Source: CAD feature listing. Evaluate the final solid. Frame: model axes, mm. A direction names the side the tool comes from. Round coordinates to 2 decimals unless told otherwise and drop trailing zeros. Order: outer loops, then holes, each group sorted by start corner. A loop starts at its lowest first (then second) coordinate and runs counter-clockwise, first axis right, second up. Notation, with made-up numbers: (56.25, -27.75) -> (105.25, -27.75) arc R28 ccw to (105.25, 11.25) -> close; hole circle Ø7 at (15, 47.5). An arc over 180 degrees is marked (long way). Answer as CSV lines item,"result".
from build123d import *

# Parameters (mm, degrees)
F2_SIZE2 = 1.3
F2_SIZE  = 0.8
F3_R     = 1.4
F4_SIZE2 = 0.5
F4_SIZE  = 2
F5_R     = 0.5


with BuildPart() as f1:
    # F0 (on Front) → F1 (revolve)
    with BuildSketch(Plane.XZ):
        Polygon((-24.5, 0), (-28.5, 0), (-28.5, -2), (-25, -2), (-25, -11), (-24.1, -11), (-24.1, -4), (-23.226406, -4), (-22.813906, -5.5), (-21.9, -5.5), (-23, -1.5), (-24.5, -1.5), align=None)
    revolve(axis=Axis((0, 0, 1.068981), (0, 0, -1)))

    # F2
    f2_edges = [f1.edges().sort_by_distance(p)[0] for p in [
        (28.5, 0, 0),
    ]]
    chamfer(f2_edges, length=F2_SIZE, length2=F2_SIZE2)

    # F3
    f3_edges = [f1.edges().sort_by_distance(p)[0] for p in [
        (25, 0, -2),
    ]]
    fillet(f3_edges, radius=F3_R)

    # F4
    f4_edges = [f1.edges().sort_by_distance(p)[0] for p in [
        (25, 0, -11),
    ]]
    chamfer(f4_edges, length=F4_SIZE, length2=F4_SIZE2)

    # F5
    f5_edges = [f1.edges().sort_by_distance(p)[0] for p in [
        (23.226406, 0, -4),
    ]]
    fillet(f5_edges, radius=F5_R)


solid = f1.part
1. Reachability of faces 4 (the cylindrical face through (-13.17, 20.66, -0.74)), 5 (the flat face through (-16.22, -18.03, -11)), 6 (the cylindrical face through (17.76, 16.29, -7.45)) from +Z, -Z, +X, -X, +Y, -Y: full face, straight path, thin tool, end or side. Return the list, or none.
Results below:
face 4,"+Z"
face 5,"-Z, +X, -X, +Y, -Y"
face 6,"-Z"
2. Mould query, pull axis X, two halves, no side actions, for faces 1 (the cylindrical face through (-23.846, 7.509, -6.239)), 2 (the flat face through (8.6, 20.4, -5.5)), 3 (the flat face through (-19, -19, -2)). Classes: released by +X, released by -X, zero draft, split by the parting line, or undercut.
Results below:
face 1,"split by the parting line"
face 2,"undercut"
face 3,"zero draft"
3. Section query C-C on z = -7.75. Return loops of the section in (x, y).
Results below:
outline,"circle Ø50 at (0, 0); hole circle Ø48.2 at (0, 0)"
4. Pin query (flat end, axial travel): pin 1 (3 mm diameter, centred on x = -12, y = 14.5, fed in from +Z); pin 2 (4 mm diameter, centred on x = -22.5, z = -10, fed in from +Y); pin 3 (3 mm diameter, centred on y = 18.5, z = -9.5, fed in from -X); pin 4 (4 mm diameter, centred on y = 15.5, z = -6, fed in from -X). Return the tip coordinate at first contact, or that it passes through.
Results below:
pin 1,"through"
pin 2,"y = 14"
pin 3,"x = -18.25"
pin 4,"x = -21.04"
5. Line query: L1, parallel to Y at x = 0, z = -7.5; L2, parallel to X at y = -18.5, z = -4.25; L3, parallel to X at y = 9.5, z = -4.5. Output: solid intervals per line, ascending. Write a range as [from, to].
Results below:
L1,"[-25, -24.1], [24.1, 25]"
L2,"[-16.82, -15.45], [-13.96, -12.35], [12.35, 13.96], [15.45, 16.82]"
L3,"[-23.12, -22.15], [-21.04, -20.04], [20.04, 21.04], [22.15, 23.12]"
